Check sheet for the drawn part. Datum: minimum x, y, z corner. Units: mm. A direction names the side the tool comes from. Give positions to 0.01 mm unless a question says otherwise; leave off trailing zeros. Write each loop counter-clockwise with the first axis right and the second up, starting at its lowest first coordinate (ties: lowest second). Pieces come first, ordered by that corner, then holes. Notation, with made-up numbers: (87, 14) -> (107, 14) arc R4 cw to (107, 19) -> close; hole circle Ø10 at (46, 39.5). An arc over 180 degrees is marked (long way). Write item = value, one per line. Start each with the question number.
1. Cross-section at A-A, the plane z = 8.9. Record the cut outline in (x, y) (3 decimals).
2. Cross-section at D-D, the plane x = 1.5. Record the cut outline in (y, z), plus the area to 3 significant figures.
3. Cross-section at C-C, the plane y = 5.5. Record the cut outline in (x, z).
4. Cross-section at B-B, the plane x = 8.9. Record the cut outline in (y, z) (3 decimals).
5. Depth check by flat-ended pin: P1, Ø6, axis at y = 3, z = 3.5, coming from the -X side; P2, Ø2, axis at x = 11, y = 3, coming from the -Z side; P3, Ø1.5, axis at x = 11, z = 14.5, coming from the +Y side; P4, Ø5, axis at x = 8.9, z = 8.9, coming from the +Y side. Enter the tip coordinate at first touch or a pass-through.
6. Mould release check, pull along X, two halves, no side actions. Record for the marked faces 1, 2 and 3: pulls with the +X half, pulls with the -X half, needs draft (parallel to the pull), parting line crosses it, or undercut.
7. Set-up check for the marked faces 4, 5 and 6: record each of +Z, -Z, +X, -X, +Y, -Y from which the full face is reachable in a straight line by a thin tool's end or side.
8. Thickness scan on line 1 along Y through (x, z) = (11.25, 1.75); line 2 along Z through (x, y) = (8.9, 10) (3 decimals); line 3 along X through (y, z) = (4.25, 8.9). Record the ranges inside material, lowest first.
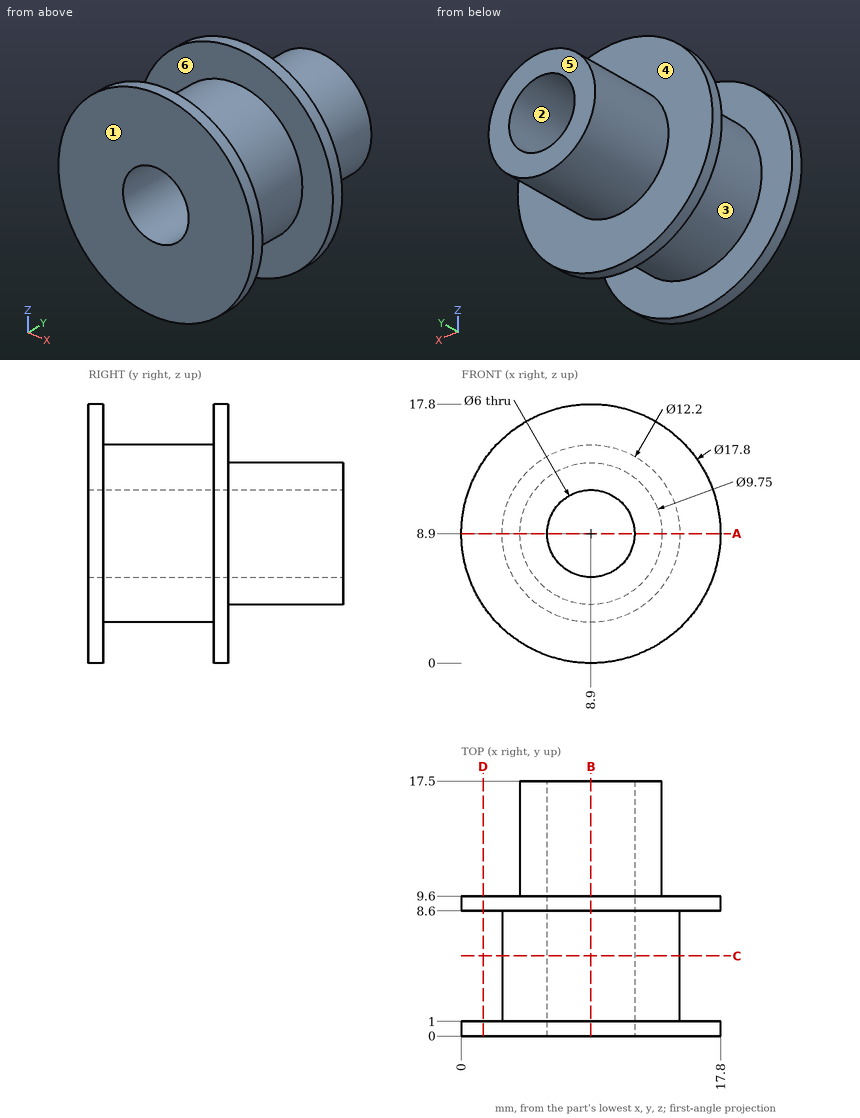
Answers:
q1.outline = (0, 0) -> (5.9, 0) -> (5.9, 17.5) -> (4.025, 17.5) -> (4.025, 9.6) -> (0, 9.6) -> (0, 8.6) -> (2.8, 8.6) -> (2.8, 1) -> (0, 1) -> close; (11.9, 0) -> (17.8, 0) -> (17.8, 1) -> (15, 1) -> (15, 8.6) -> (17.8, 8.6) -> (17.8, 9.6) -> (13.775, 9.6) -> (13.775, 17.5) -> (11.9, 17.5) -> close
q2.outline = (0, 3.96) -> (1, 3.96) -> (1, 13.84) -> (0, 13.84) -> close; (8.6, 3.96) -> (9.6, 3.96) -> (9.6, 13.84) -> (8.6, 13.84) -> close
q2.area = 19.8 mm^2
q3.outline = circle Ø12.2 at (8.9, 8.9); hole circle Ø6 at (8.9, 8.9)
q4.outline = (0, 0) -> (1, 0) -> (1, 2.8) -> (8.6, 2.8) -> (8.6, 0) -> (9.6, 0) -> (9.6, 4.025) -> (17.5, 4.025) -> (17.5, 5.9) -> (0, 5.9) -> close; (0, 11.9) -> (17.5, 11.9) -> (17.5, 13.775) -> (9.6, 13.775) -> (9.6, 17.8) -> (8.6, 17.8) -> (8.6, 15) -> (1, 15) -> (1, 17.8) -> (0, 17.8) -> close
q5.P1 = 0.58
q5.P2 = 2.9
q5.P3 = 9.6
q5.P4 = through
q6.face_1 = needs draft
q6.face_2 = undercut
q6.face_3 = parting line crosses it
q7.face_4 = +Y
q7.face_5 = +Z, -Z, +X, -X, +Y
q7.face_6 = none
q8.line_1 = 0 to 1, 8.6 to 9.6
q8.line_2 = 4.025 to 5.9, 11.9 to 13.775
q8.line_3 = 2.8 to 5.9, 11.9 to 15
